Part model, mm, in its own coordinate system. Round coordinates to 2 decimals unless told otherwise and drop trailing zeros. Write each loop counter-clockwise with the first axis right and the second up, starting at its lowest first coordinate (ties: lowest second). Pieces come first, ordered by that corner, then holes. Notation, with made-up numbers: M -33.75,-15.5 L 10.25,-15.5 A19 cw 10.25,-3.5 Z; hole C -2.75,75 d9. An arc over 180 degrees is marked long. Answer as a JSON object with one key per item and string values. Group by question number.
1. Band-saw the part on C-C, the plane z = 0.85. Write the cut outline in (x, y) (3 decimals), plus the area to 3 significant figures.
2. Drill centre lines: line 1 (Y direction, x = 155.75, z = 1); line 2 (X direction, y = 40, z = 0.2); line 3 (Y direction, x = 160.5, z = 1.4). Where is each one in solid material? Low to high. Write a range as from..to.
3. Two-plate mould, pull along Y, no slides. Class faces 1 (the face through (167.976, 17.277, 1.479)), 2 (the face through (159, 18, 0)), 3 (the face through (156.7, 39.9, 1.5)): +Y half, -Y half, draft (parallel to the pull), parting line (faces both ways), or undercut.
4. Drop flat-ended pins along their axis: pin 1 (2.5 mm diameter, centred on x = 154.87, y = 39.1, fed in from -Z); pin 2 (1 mm diameter, centred on y = 31.5, z = 1, fed in from -X). Give the stop position or say it passes through.
5. Band-saw the part on A-A, the plane y = 25. Write the cut outline in (x, z) (3 decimals).
6. Band-saw the part on D-D, the plane y = 1.5. Write the cut outline in (x, z), plus the area to 3 significant figures.
7. Band-saw the part on B-B, the plane x = 159.5. Write the cut outline in (y, z).
Autodesk Inventor part; units mm, degrees
ref_plane "YZ Plane" through (0, 0, 0) normal (1, 0, 0) x (0, 1, 0)
ref_plane "XZ Plane" through (0, 0, 0) normal (0, 1, 0) x (-1, 0, 0)
ref_plane "XY Plane" through (0, 0, 0) normal (0, 0, 1) x (1, 0, 0)
sketch "スケッチ1" plane through (0, 0, 0) normal (0, 0, 1) x (1, 0, 0)
  circle A0 centre (154.8697, 39.0954) radius 2
  circle A1 centre (153.5524, -4.4926) radius 2
  circle A2 centre (160, 25) radius 2
  circle A3 centre (154.8697, 39.0954) radius 4
  circle A4 centre (153.5524, -4.4926) radius 4
  circle A5 centre (160, 25) radius 7
  circle A6 centre (160, 25) radius 5.025
  arc A7 (149.7263, -3.3259) -> (150.9802, 38.1619) centre (74.1465, 19.7211) ccw
  arc A8 (156.1251, -7.5554) -> (157.6227, 41.9973) centre (134.7514, 17.8895) ccw
  point P0 (0, 0)
  point P1 (0, 0)
  dimension "d0" = 8
  dimension "d1" = 8
  dimension "d2" = 14
  dimension "d3" = 10.05
extrude "押し出し1" add sketch "スケッチ1" along normal blind 3 contours A3 | A3 A8 A5 A7 | A8 A4 A7 A5 | A5 | A4
properties part number "原動節固定部" material "アルミニウム 2014-T4"
Worked answers:
{
 "1": {"outline": "M 149.726,-3.326 A4 ccw 156.125,-7.555 A33.231 ccw 157.623,41.997 A4 ccw 150.98,38.162 A79.017 cw Z; hole C 153.552,-4.493 d4; hole C 154.87,39.095 d4; hole C 160,25 d10.05", "area": "529 mm^2"},
 "2": {"line 1": "y = -7.83..22.32, 27.68..37.3, 40.89..43", "line 2": "x = 150.97..153.09, 156.65..159.56", "line 3": "y = -3.12..20, 30..38.9"},
 "3": {"face 1": "parting line", "face 2": "draft", "face 3": "undercut"},
 "4": {"pin 1": "passes through", "pin 2": "stops at x = 152.2"},
 "5": {"outline": "M 152.986,0 L 154.975,0 L 154.975,3 L 152.986,3 Z; M 165.025,0 L 167.212,0 L 167.212,3 L 165.025,3 Z"},
 "6": {"outline": "M 151.03,0 L 163.66,0 L 163.66,3 L 151.03,3 Z", "area": "37.9 mm^2"},
 "7": {"outline": "M -4.29,0 L 20,0 L 20,3 L -4.29,3 Z; M 30,0 L 40.07,0 L 40.07,3 L 30,3 Z"}
}
